Input: part model. Units: mm. Frame: model coordinates. A direction names the side the tool comes from. Round coordinates to 2 decimals unless told otherwise and drop trailing zeros. Order: outer loops, then holes, each group sorted by start corner. A loop starts at its lowest first (then second) coordinate and runs counter-clockwise, first axis right, second up. Notation, with made-up numbers: (55.5, 21) - (112.5, 21) arc R8 cw to (112.5, 35) - close; hole circle Ø1 at (69, -9.5). An arc over 180 degrees is marked (long way). One line per item, written item: value. Start each with the question number.
from build123d import *

# Parameters (mm, degrees)
CROQUIS1_W              = 320
CROQUIS1_H              = 437
SALIENTE_EXTRUIR1_DEPTH = 1.5
CROQUIS2_W              = 317
CROQUIS2_H              = 434
SALIENTE_EXTRUIR2_DEPTH = 135
CORTAR_EXTRUIR1_DEPTH   = 1.5
CORTAR_EXTRUIR2_DEPTH   = 1.5
CROQUIS6_R              = 2.5
CORTAR_EXTRUIR4_DEPTH   = 320


with BuildPart() as part:
    # Croquis1 → Saliente-Extruir1 (new body)
    with BuildSketch(Plane.XY):
        with Locations((-160, 218.5)):
            Rectangle(CROQUIS1_W, CROQUIS1_H)
    extrude(amount=SALIENTE_EXTRUIR1_DEPTH)

    # Croquis2 → Saliente-Extruir2 (add)
    with BuildSketch(Plane.XY):
        Polygon((0, 436), (0, 437), (-1, 437), (-319, 437), (-320, 437), (-320, 436), (-320, 1), (-320, 0), (-319, 0), (-1, 0), (0, 0), (0, 1), align=None)
        with Locations((-160, 218.5)):
            Rectangle(CROQUIS2_W, CROQUIS2_H, mode=Mode.SUBTRACT)
    extrude(amount=SALIENTE_EXTRUIR2_DEPTH)

    # Croquis3 → Cortar-Extruir1 (cut)
    with BuildSketch(Plane.XZ):
        with BuildLine():
            Line((-247.5, 95), (-247.5, 135))
            Line((-247.5, 135), (-227.5, 135))
            Line((-227.5, 135), (-227.5, 95))
            ThreePointArc((-227.5, 95), (-237.5, 85), (-247.5, 95))
        make_face()
        with BuildLine():
            Line((-92.5, 95), (-92.5, 135))
            Line((-92.5, 135), (-72.5, 135))
            Line((-72.5, 135), (-72.5, 95))
            ThreePointArc((-72.5, 95), (-82.5, 85), (-92.5, 95))
        make_face()
    extrude(amount=-CORTAR_EXTRUIR1_DEPTH, mode=Mode.SUBTRACT)

    # Croquis4 → Cortar-Extruir2 (cut)
    with BuildSketch(Plane.XZ):
        with BuildLine():
            Line((-305, 95), (-305, 135))
            Line((-305, 135), (-265, 135))
            Line((-265, 135), (-265, 95))
            ThreePointArc((-265, 95), (-285, 75), (-305, 95))
        make_face()
    extrude(amount=-CORTAR_EXTRUIR2_DEPTH, mode=Mode.SUBTRACT)

    # Croquis6 → Cortar-Extruir4 (cut)
    with BuildSketch(Plane.ZY.offset(320)):
        with Locations((125, 368.5)):
            Circle(CROQUIS6_R)
        with Locations((125, 68.5)):
            Circle(CROQUIS6_R)
        with Locations((125, 218.5)):
            Circle(CROQUIS6_R)
    extrude(amount=-CORTAR_EXTRUIR4_DEPTH, mode=Mode.SUBTRACT)


solid = part.part
Item 1: Line query: L1, parallel to Y at x = -0.4, z = 125; L2, parallel to X at y = 294.5, z = 62.5; L3, parallel to Y at x = -180.5, z = 71.5. Output: solid intervals per line, ascending.
Item 2: Section query C-C on z = 44.5. Return loops of the section in (x, y).
Item 3: Section query B-B on y = 59. Return loops of the section in (x, z), and give its area (4 significant figures).
Item 4: First-contact query: pin 1 Ø3 at (y, z) = (218.5, 125) entering from -X; pin 2 Ø3 at (x, y) = (-120, 142) entering from +Z; pin 3 Ø8 at (x, z) = (-154.5, 106.5) entering from -Y. Flat tips, straight axial feed; report the tip coordinate or a pass-through.
Item 5: Pull-direction query (X, two-part tool) for faces 4 (the face through (0, 215, 67)), 5 (the face through (-162, 437, 67)), 6 (the face through (-82.3, 0.7, 85)); classes: released by +X, released by -X, zero draft, split by the parting line, or undercut.
Item 6: Reachability of faces 1 (the face through (-162, 1.5, 52)), 2 (the face through (-285, 1, 75)), 3 (the face through (-320, 215, 67)) from +Z, -Z, +X, -X, +Y, -Y: full face, straight path, thin tool, end or side. Return the list, or none.
Item 7: Section query A-A on x = -237.5. Return loops of the section in (y, z).
Geometry results:
1. L1: y = 0 to 66, 71 to 216, 221 to 366, 371 to 437
1. L2: x = -320 to -318.5, -1.5 to 0
1. L3: y = 0 to 1.5, 435.5 to 437
2. outline: (-320, 0) - (0, 0) - (0, 437) - (-320, 437) - close; hole (-318.5, 1.5) - (-1.5, 1.5) - (-1.5, 435.5) - (-318.5, 435.5) - close
3. outline: (-320, 0) - (0, 0) - (0, 135) - (-1.5, 135) - (-1.5, 1.5) - (-318.5, 1.5) - (-318.5, 135) - (-320, 135) - close
3. area: 880.5 mm^2
4. pin 1: passes through
4. pin 2: stops at z = 1.5
4. pin 3: stops at y = 0
5. face 4: released by +X
5. face 5: zero draft
5. face 6: undercut
6. face 1: +Z
6. face 2: +Z, -Y
6. face 3: +Z, -Z, -X, +Y, -Y
7. outline: (0, 0) - (437, 0) - (437, 135) - (435.5, 135) - (435.5, 1.5) - (1.5, 1.5) - (1.5, 85) - (0, 85) - close
